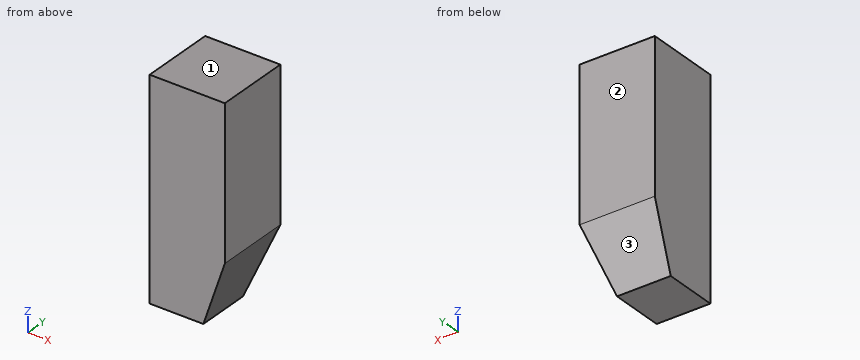
from build123d import *

# Parameters (mm, degrees)
F0_W     = 44.45
F0_H     = 44.45
F1_DEPTH = 254
F2_SIZE2 = 76.2
F2_SIZE  = 25.4
F3_SIZE2 = 76.2
F3_SIZE  = 25.4


with BuildPart() as f1:
    # F0 (on Top) → F1 (new body)
    with BuildSketch(Plane.XY):
        with Locations((-22.225, 22.225)):
            Rectangle(F0_W, F0_H)
        with Locations((22.225, 22.225)):
            Rectangle(F0_W, F0_H)
        with Locations((22.225, -22.225)):
            Rectangle(F0_W, F0_H)
        with Locations((-22.225, -22.225)):
            Rectangle(F0_W, F0_H)
    extrude(amount=F1_DEPTH)

    # F2
    f2_edges = [f1.edges().sort_by_distance(p)[0] for p in [
        (44.45, 0, 0),
    ]]
    f2_side = f1.faces().sort_by_distance((0, 0, 0))[0]
    chamfer(f2_edges, length=F2_SIZE, length2=F2_SIZE2, reference=f2_side)

    # F3
    f3_edges = [f1.edges().sort_by_distance(p)[0] for p in [
        (-12.7, 44.45, 0),
    ]]
    f3_side = f1.faces().sort_by_distance((-12.7, 0, 0))[0]
    chamfer(f3_edges, length=F3_SIZE, length2=F3_SIZE2, reference=f3_side)


solid = f1.part
Build history of the part. All positions in model axes, mm. Face numbers are marked on the shaded views. Coordinates: 2 decimals unless noted, no trailing zeros. Order: outer loops, then holes, each group sorted by start corner. A loop starts at its lowest first (then second) coordinate and runs counter-clockwise, first axis right, second up. Notation, with made-up numbers: (22, 78.5) - (30, 78.5) arc R17 cw to (30, 90.5) - close; hole circle Ø1 at (-34, 52.25). An arc over 180 degrees is marked (long way). Write each question's results on one line, items separated by ' | '. Start each with the question number.
Item 1: Wall check: probe 1 along X at (y, z) = (-32.5, 27.5); probe 2 along Y at (x, z) = (34.5, 65); probe 3 along X at (y, z) = (15, 32). Give the ranges that are in metal, low to high. Write a range as [from, to].
Item 2: Band-saw the part on C-C on z = 24.5. Write the cut outline in (x, y).
Item 3: Band-saw the part on A-A on y = -19.5. Write the cut outline in (x, z).
Item 4: Mould opens along Z. For the marked faces 1, 2 and 3 say: released by +Z, released by -Z, zero draft, split by the parting line, or undercut.
Item 5: Band-saw the part on D-D on z = 64. Write the cut outline in (x, y).
Item 6: Flat gauge pins, fed straight in: pin 1 (8 mm diameter, centred on y = -25, z = 73.5, fed in from +X); pin 2 (12 mm diameter, centred on y = -31.5, z = 33, fed in from +X). Where does each tip first touch, or does it go through?
Numbers:
1) probe 1: [-44.45, 28.22] | probe 2: [-44.45, 40.72] | probe 3: [-44.45, 29.72]
2) outline: (-44.45, -44.45) - (27.22, -44.45) - (27.22, 27.22) - (-44.45, 27.22) - close
3) outline: (-44.45, 0) - (19.05, 0) - (44.45, 76.2) - (44.45, 254) - (-44.45, 254) - close
4) face 1: released by +Z | face 2: zero draft | face 3: released by -Z
5) outline: (-44.45, -44.45) - (40.38, -44.45) - (40.38, 40.38) - (-44.45, 40.38) - close
6) pin 1: x = 44.45 | pin 2: x = 32.05
